```python
from build123d import *

# Parameters (mm, degrees)
EXTRUDE_1_DEPTH = 3
FILLET_1_R      = 2


with BuildPart() as part:
    # 草图1 → 凸台-拉伸1 (new body)
    with BuildSketch(Plane.XY):
        with BuildLine():
            Line((7.125, 20.5), (-7.125, 20.5))
            Line((-7.125, 20.5), (-7.125, 10.5))
            Line((-7.125, 10.5), (-4.025, 10.5))
            ThreePointArc((-4.025, 10.5), (-3.314357685, 10.205642315), (-3.02, 9.495))
            ThreePointArc((-3.02, 9.495), (-3.314357685, 8.784357685), (-4.025, 8.49))
            Line((-4.025, 8.49), (-4.025, 5.51))
            ThreePointArc((-4.025, 5.51), (-3.314357685, 5.215642315), (-3.02, 4.505))
            ThreePointArc((-3.02, 4.505), (-3.314357685, 3.794357685), (-4.025, 3.5))
            Line((-4.025, 3.5), (-7.125, 3.5))
            Line((-7.125, 3.5), (-7.125, -3.5))
            Line((-7.125, -3.5), (-4.025, -3.5))
            ThreePointArc((-4.025, -3.5), (-3.314357685, -3.794357685), (-3.02, -4.505))
            ThreePointArc((-3.02, -4.505), (-3.314357685, -5.215642315), (-4.025, -5.51))
            Line((-4.025, -5.51), (-4.025, -8.49))
            ThreePointArc((-4.025, -8.49), (-3.314357685, -8.784357685), (-3.02, -9.495))
            ThreePointArc((-3.02, -9.495), (-3.314357685, -10.205642315), (-4.025, -10.5))
            Line((-4.025, -10.5), (-7.125, -10.5))
            Line((-7.125, -10.5), (-7.125, -20.5))
            Line((-7.125, -20.5), (7.125, -20.5))
            Line((7.125, -20.5), (7.125, -11.830127019))
            Line((7.125, -11.830127019), (4.625, -7.5))
            Line((4.625, -7.5), (4.625, 7.5))
            Line((4.625, 7.5), (7.125, 11.830127019))
            Line((7.125, 11.830127019), (7.125, 20.5))
        make_face()
        with BuildLine():
            Line((2.115, -17.55), (-0.165, -17.55))
            ThreePointArc((-0.165, -17.55), (-1.17, -18.555), (-2.175, -17.55))
            Line((-2.175, -17.55), (-2.175, -14.45))
            ThreePointArc((-2.175, -14.45), (-1.17, -13.445), (-0.165, -14.45))
            Line((-0.165, -14.45), (2.115, -14.45))
            ThreePointArc((2.115, -14.45), (3.12, -13.445), (4.125, -14.45))
            Line((4.125, -14.45), (4.125, -17.55))
            ThreePointArc((4.125, -17.55), (3.12, -18.555), (2.115, -17.55))
        make_face(mode=Mode.SUBTRACT)
        with BuildLine():
            Line((2.115, 14.45), (-0.165, 14.45))
            ThreePointArc((-0.165, 14.45), (-1.17, 13.445), (-2.175, 14.45))
            Line((-2.175, 14.45), (-2.175, 17.55))
            ThreePointArc((-2.175, 17.55), (-1.17, 18.555), (-0.165, 17.55))
            Line((-0.165, 17.55), (2.115, 17.55))
            ThreePointArc((2.115, 17.55), (3.12, 18.555), (4.125, 17.55))
            Line((4.125, 17.55), (4.125, 14.45))
            ThreePointArc((4.125, 14.45), (3.12, 13.445), (2.115, 14.45))
        make_face(mode=Mode.SUBTRACT)
    extrude(amount=EXTRUDE_1_DEPTH)

    # 圆角1
    fillet_1_edges = [part.edges().sort_by_distance(p)[0] for p in [
        (-7.125, 20.5, 1.5),
        (7.125, 20.5, 1.5),
        (7.125, -20.5, 1.5),
        (-7.125, -20.5, 1.5),
    ]]
    fillet(fillet_1_edges, radius=FILLET_1_R)


solid = part.part
```
Check sheet for the modelled part. Datum: model origin and axes. Units: mm. A direction names the side the tool comes from. Give positions to 0.01 mm unless a question says otherwise; leave off trailing zeros. Write each loop counter-clockwise with the first axis right and the second up, starting at its lowest first coordinate (ties: lowest second). Pieces come first, ordered by that corner, then holes.
Item 1: Access from +Z, -Z, +X, -X, +Y, -Y to the whole of each face (thin tool, end or side, straight path). Record for faces 1 (the face through (1, -14.45, 1)), 2 (the face through (-6, 10.5, 1)), 3 (the face through (-7.125, -14, 1)), 4 (the face through (5.892, -9.695, 1.479)), 5 (the face through (7.125, -15, 1)).
Item 2: Cross-section at C-C (z = 1.9). Count the separate pieces of the cut face and the enclosed holes in it, and give its area (3 significant figures).
Item 3: Cross-section at B-B (y = -16.5). Enter the section's corners in (x, z) (3 decimals).
Item 4: Gauge pin test, flat end, axial feed: pin 1 (0.9 mm diameter, centred on y = 7, z = 2, fed in from -X) (3 decimals). Record the tip position at first contact, or that the pin passes through.
Item 5: Cross-section at A-A (x = 1.5). Enter the section's corners in (y, z).
Item 6: Draft check along Y on faces 6 (the face through (6.524, 19.93, 1.521)), 7 (the face through (1, 14.45, 1)), 8 (the face through (7.125, 15, 1)), 9 (the face through (5.858, 9.635, 1.479)). Enter one of: released by +Y, released by -Y, zero draft, split by the parting line, or undercut.
Item 7: Scan lines: L1, parallel to Y at x = 0.25, z = 0.65; L2, parallel to Y at x = 3.5, z = 2.15; L3, parallel to X at y = 17, z = 0.2 (3 decimals). Record each from-to range of solid material in increasing order.
Item 8: Cross-section at D-D (x = -1.17). Enter the section's corners in (y, z) (3 decimals), and give its area (3 significant figures).
Report:
1. face 1: +Z, -Z
1. face 2: +Z, -Z, -X
1. face 3: +Z, -Z, -X, +Y, -Y
1. face 4: +Z, -Z, +X
1. face 5: +Z, -Z, +X, +Y, -Y
2. separate pieces: 1
2. enclosed holes: 2
2. area: 431 mm2
3. outline: (-7.125, 0) - (-2.175, 0) - (-2.175, 3) - (-7.125, 3) - close; (4.125, 0) - (7.125, 0) - (7.125, 3) - (4.125, 3) - close
4. pin 1: stops at x = -4.025
5. outline: (-20.5, 0) - (-17.55, 0) - (-17.55, 3) - (-20.5, 3) - close; (-14.45, 0) - (14.45, 0) - (14.45, 3) - (-14.45, 3) - close; (17.55, 0) - (20.5, 0) - (20.5, 3) - (17.55, 3) - close
6. face 6: released by +Y
6. face 7: undercut
6. face 8: zero draft
6. face 9: undercut
7. L1: y = -20.5 to -17.55, -14.45 to 14.45, 17.55 to 20.5
7. L2: y = -20.5 to -18.48, -13.52 to 13.52, 18.48 to 20.5
7. L3: x = -7.125 to -2.175, 4.125 to 7.125
8. outline: (-20.5, 0) - (-18.555, 0) - (-18.555, 3) - (-20.5, 3) - close; (-13.445, 0) - (13.445, 0) - (13.445, 3) - (-13.445, 3) - close; (18.555, 0) - (20.5, 0) - (20.5, 3) - (18.555, 3) - close
8. area: 92.3 mm2
